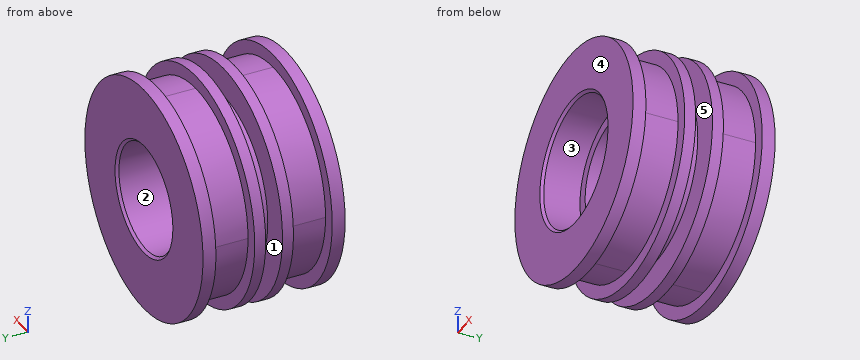
```python
from build123d import *

# Parameters (mm, degrees)
SKETCH1_R           = 44.175
BOSS_EXTRUDE1_DEPTH = 27.5
SKETCH3_W           = 11
SKETCH3_H           = 6.5
SKETCH4_W           = 5
SKETCH4_H           = 15
SKETCH9_R           = 20.625
CUT_EXTRUDE2_DEPTH  = 84.233774695
CHAMFER1_SIZE       = 1
SKETCH10_R          = 24.5
CUT_EXTRUDE3_DEPTH  = 15
CHAMFER2_SIZE       = 1


with BuildPart() as part:
    # Sketch1 → Boss-Extrude1 (new, symmetric)
    with BuildSketch(Plane(origin=(0, 0, 0), x_dir=(1, 0, 0), z_dir=(0, 1, 0))):
        with Locations(Location((0, 0, 0), (0, 0, 270))):
            Circle(SKETCH1_R)
    extrude(amount=BOSS_EXTRUDE1_DEPTH, both=True)

    # Cut-Sweep1: sweep along a curve in space
    with BuildLine() as cut_sweep1_path:
        ThreePointArc((0, 27.5, 44.175), (31.236442059, 27.5, 31.236442059), (44.175, 27.5, 0))
        ThreePointArc((44.175, 27.5, 0), (31.236442059, 27.5, -31.236442059), (0, 27.5, -44.175))
        ThreePointArc((0, 27.5, -44.175), (-31.236442059, 27.5, -31.236442059), (-44.175, 27.5, 0))
        ThreePointArc((-44.175, 27.5, 0), (-31.236442059, 27.5, 31.236442059), (0, 27.5, 44.175))
    # Sketch3 → Cut-Sweep1 (sweep, cut)
    with BuildSketch(Plane.XY):
        with Locations((38.675, 0)):
            Rectangle(SKETCH3_W, SKETCH3_H)
    sweep(path=cut_sweep1_path.line, mode=Mode.SUBTRACT)

    # Cut-Sweep2: sweep along a curve in space
    with BuildLine() as cut_sweep2_path:
        ThreePointArc((0, 27.5, 44.175), (31.236442059, 27.5, 31.236442059), (44.175, 27.5, 0))
        ThreePointArc((44.175, 27.5, 0), (31.236442059, 27.5, -31.236442059), (0, 27.5, -44.175))
        ThreePointArc((0, 27.5, -44.175), (-31.236442059, 27.5, -31.236442059), (-44.175, 27.5, 0))
        ThreePointArc((-44.175, 27.5, 0), (-31.236442059, 27.5, 31.236442059), (0, 27.5, 44.175))
    # Sketch4 → Cut-Sweep2 (sweep, cut)
    with BuildSketch(Plane.XY):
        with Locations((41.675, 15)):
            Rectangle(SKETCH4_W, SKETCH4_H)
    cut_sweep2 = sweep(path=cut_sweep2_path.line, mode=Mode.SUBTRACT)

    # Mirror1: Cut-Sweep2 across plane
    add(cut_sweep2.mirror(Plane.ZX), mode=Mode.SUBTRACT)

    # Sketch9 → Cut-Extrude2 (cut, through all)
    with BuildSketch(Plane(origin=(0, 27.5, 0), x_dir=(1, 0, 0), z_dir=(0, 1, 0))):
        with Locations(Location((0, 0, 0), (0, 0, 270))):
            Circle(SKETCH9_R)
    extrude(amount=-CUT_EXTRUDE2_DEPTH, mode=Mode.SUBTRACT)

    # Chamfer1
    chamfer1_edges = [part.edges().sort_by_distance(p)[0] for p in [
        (0, 27.5, -20.625),
    ]]
    chamfer(chamfer1_edges, length=CHAMFER1_SIZE)

    # Sketch10 → Cut-Extrude3 (cut)
    with BuildSketch(Plane.XZ.offset(27.5)):
        with Locations(Location((0, 0, 0), (0, 0, 270))):
            Circle(SKETCH10_R)
    extrude(amount=-CUT_EXTRUDE3_DEPTH, mode=Mode.SUBTRACT)

    # Chamfer2
    chamfer2_edges = [part.edges().sort_by_distance(p)[0] for p in [
        (0, -27.5, 24.5),
    ]]
    chamfer(chamfer2_edges, length=CHAMFER2_SIZE)


solid = part.part
```
Source: CAD feature listing. Evaluate the final solid. Frame: model axes, mm. Face numbers are marked on the shaded views. A direction names the side the tool comes from. Give positions to 0.01 mm unless a question says otherwise; leave off trailing zeros. Write each loop counter-clockwise with the first axis right and the second up, starting at its lowest first coordinate (ties: lowest second). Pieces come first, ordered by that corner, then holes.
1. Access query for the marked faces 3, 4 and 5. Directions: +Z, -Z, +X, -X, +Y, -Y. A direction counts if a zero-diameter tool reaches every point of the face in a straight line with its end or side. Return the directions, or none.
2. First-contact query: pin 1 (6 mm diameter, centred on y = 21, z = 12.5, fed in from -X); pin 2 (4 mm diameter, centred on y = 19, z = -18.5, fed in from +X); pin 3 (10 mm diameter, centred on y = -15, z = 25.5, fed in from -X). Flat tips, straight axial feed; report the tip coordinate or a pass-through.
3. Section query D-D (z = -31.5). Return the cut outline in (x, y).
4. Section query A-A (z = 36). Return the cut outline in (x, y), then the cut area to 3 significant figures.
5. Pull-direction query (X, two-part tool) for the marked faces 1 and 2; classes: +X half, -X half, draft (parallel to the pull), parting line (faces both ways), or undercut.
6. Section query C-C (z = 27). Return the cut outline in (x, y), then the cut area to 3 significant figures.
7. Material intervals for line 1 along Y through (x, z) = (13, -37.5); line 2 along X through (y, z) = (13, 0) (3 decimals); line 3 along X through (y, z) = (-16, 0) (3 decimals), sorted ascending.
8. Section query B-B (y = -9). Return the cut outline in (x, z) (3 decimals).
Output values:
1. face 3: -Y
1. face 4: +Z, -Z, +X, -X, -Y
1. face 5: none
2. pin 1: stops at x = -43.05
2. pin 2: stops at x = 35.53
2. pin 3: stops at x = -33.38
3. outline: (-30.97, -27.5) - (30.97, -27.5) - (30.97, -22.5) - (23.29, -22.5) - (23.29, -7.5) - (30.97, -7.5) - (30.97, -3.25) - (10.41, -3.25) - (10.41, 3.25) - (30.97, 3.25) - (30.97, 7.5) - (23.29, 7.5) - (23.29, 22.5) - (30.97, 22.5) - (30.97, 27.5) - (-30.97, 27.5) - (-30.97, 22.5) - (-23.29, 22.5) - (-23.29, 7.5) - (-30.97, 7.5) - (-30.97, 3.25) - (-10.41, 3.25) - (-10.41, -3.25) - (-30.97, -3.25) - (-30.97, -7.5) - (-23.29, -7.5) - (-23.29, -22.5) - (-30.97, -22.5) - close
4. outline: (-25.6, -27.5) - (25.6, -27.5) - (25.6, -22.5) - (15.45, -22.5) - (15.45, -7.5) - (25.6, -7.5) - (25.6, -3.25) - (-25.6, -3.25) - (-25.6, -7.5) - (-15.45, -7.5) - (-15.45, -22.5) - (-25.6, -22.5) - close; (-25.6, 3.25) - (25.6, 3.25) - (25.6, 7.5) - (15.45, 7.5) - (15.45, 22.5) - (25.6, 22.5) - (25.6, 27.5) - (-25.6, 27.5) - (-25.6, 22.5) - (-15.45, 22.5) - (-15.45, 7.5) - (-25.6, 7.5) - close
4. area: 1,870 mm2
5. face 1: draft
5. face 2: undercut
6. outline: (-34.96, -27.5) - (34.96, -27.5) - (34.96, -22.5) - (28.38, -22.5) - (28.38, -7.5) - (34.96, -7.5) - (34.96, -3.25) - (19.28, -3.25) - (19.28, 3.25) - (34.96, 3.25) - (34.96, 7.5) - (28.38, 7.5) - (28.38, 22.5) - (34.96, 22.5) - (34.96, 27.5) - (-34.96, 27.5) - (-34.96, 22.5) - (-28.38, 22.5) - (-28.38, 7.5) - (-34.96, 7.5) - (-34.96, 3.25) - (-19.28, 3.25) - (-19.28, -3.25) - (-34.96, -3.25) - (-34.96, -7.5) - (-28.38, -7.5) - (-28.38, -22.5) - (-34.96, -22.5) - close
6. area: 3,250 mm2
7. line 1: y = -27.5 to -22.5, -7.5 to -3.25, 3.25 to 7.5, 22.5 to 27.5
7. line 2: x = -39.175 to -20.625, 20.625 to 39.175
7. line 3: x = -39.175 to -24.5, 24.5 to 39.175
8. outline: circle Ø78.35 at (0, 0); hole circle Ø41.25 at (0, 0)
